Geometry: final body of the model. Coordinates: model frame, mm. A direction names the side the tool comes from. Coordinates: 2 decimals unless noted, no trailing zeros. Order: outer loops, then holes, each group sorted by start corner. A loop starts at its lowest first (then second) coordinate and runs counter-clockwise, first axis right, second up. Notation, with made-up numbers: (-36.5, 45) -> (-16.5, 45) arc R12 cw to (-16.5, 51) -> close; hole circle Ø9 at (63.5, 67.5). An arc over 180 degrees is marked (long way). Use CSV: the item, a comma, the result in double quotes. Start each with the question number.
from build123d import *

# Parameters (mm, degrees)
BOSS_EXTRUDE1_DEPTH = 1.3
BOSS_EXTRUDE3_DEPTH = 3
CUT_EXTRUDE1_DEPTH  = 3
SKETCH11_W          = 6.5
SKETCH11_H          = 9
CUT_EXTRUDE2_DEPTH  = 4.3
SKETCH12_W          = 12.1
SKETCH12_H          = 12.1
CUT_EXTRUDE4_DEPTH  = 1.3
SKETCH17_W          = 14.5
SKETCH17_H          = 14.3
SKETCH17_W_2        = 12.1
SKETCH17_H_2        = 12.1
BOSS_EXTRUDE4_DEPTH = 6.25
CUT_EXTRUDE5_DEPTH  = 4.3
BOSS_EXTRUDE5_DEPTH = 6.25
CUT_EXTRUDE6_START  = -3
CUT_EXTRUDE6_DEPTH  = 23
SKETCH21_W          = 2.5
SKETCH21_H          = 2.5
CUT_EXTRUDE7_DEPTH  = 10
BOSS_EXTRUDE7_DEPTH = 7.6
SKETCH25_W          = 2
SKETCH25_H          = 2
BOSS_EXTRUDE8_DEPTH = 7.6
SKETCH27_W          = 1
SKETCH27_H          = 18.4
CUT_EXTRUDE8_DEPTH  = 7.5
FILLET1_R           = 0.4


with BuildPart() as part:
    # Sketch1 → Boss-Extrude1 (new body)
    with BuildSketch(Plane.XY):
        with BuildLine():
            Line((2.7, 0), (52.9, 0))
            ThreePointArc((52.9, 0), (54.809188309, 0.790811691), (55.6, 2.7))
            Line((55.6, 2.7), (55.6, 19.4))
            ThreePointArc((55.6, 19.4), (54.809188309, 21.309188309), (52.9, 22.1))
            Line((52.9, 22.1), (2.7, 22.1))
            ThreePointArc((2.7, 22.1), (0.790811691, 21.309188309), (0, 19.4))
            Line((0, 19.4), (0, 2.7))
            ThreePointArc((0, 2.7), (0.790811691, 0.790811691), (2.7, 0))
        make_face()
    extrude(amount=BOSS_EXTRUDE1_DEPTH)

    # Sketch4 → Boss-Extrude3 (add)
    with BuildSketch(Plane.XY.offset(1.3)):
        with BuildLine():
            Line((54.25, 2.85), (54.25, 19.25))
            ThreePointArc((54.25, 19.25), (53.810660172, 20.310660172), (52.75, 20.75))
            Line((52.75, 20.75), (2.85, 20.75))
            ThreePointArc((2.85, 20.75), (1.789339828, 20.310660172), (1.35, 19.25))
            Line((1.35, 19.25), (1.35, 2.85))
            ThreePointArc((1.35, 2.85), (1.789339828, 1.789339828), (2.85, 1.35))
            Line((2.85, 1.35), (52.75, 1.35))
            ThreePointArc((52.75, 1.35), (53.810660172, 1.789339828), (54.25, 2.85))
        make_face()
    extrude(amount=BOSS_EXTRUDE3_DEPTH)

    # Sketch5 → Cut-Extrude1 (cut)
    with BuildSketch(Plane.XY.offset(4.3)):
        with BuildLine():
            Line((51.75, 18.75), (3.85, 18.75))
            ThreePointArc((3.85, 18.75), (3.496446609, 18.603553391), (3.35, 18.25))
            Line((3.35, 18.25), (3.35, 3.85))
            ThreePointArc((3.35, 3.85), (3.496446609, 3.496446609), (3.85, 3.35))
            Line((3.85, 3.35), (51.75, 3.35))
            ThreePointArc((51.75, 3.35), (52.103553391, 3.496446609), (52.25, 3.85))
            Line((52.25, 3.85), (52.25, 18.25))
            ThreePointArc((52.25, 18.25), (52.103553391, 18.603553391), (51.75, 18.75))
        make_face()
    extrude(amount=-CUT_EXTRUDE1_DEPTH, mode=Mode.SUBTRACT)

    # Sketch10 → Cut-Revolve1 (revolve, cut)
    with BuildSketch(Plane(origin=(0, 20.75, 0), x_dir=(1, 0, 0), z_dir=(0, 1, 0))):
        with BuildLine():
            Line((40.35, -2), (40.35, -3.6))
            ThreePointArc((40.35, -3.6), (39.55, -2.8), (40.35, -2))
        make_face()
    cut_revolve1 = revolve(axis=Axis((40.35, 20.75, 2), (0, 0, 1)), mode=Mode.SUBTRACT)

    # Mirror1: Cut-Revolve1 across plane
    add(cut_revolve1.mirror(Plane(origin=(0, 11.05, 0), x_dir=(0, 0, 1), z_dir=(0, -1, 0))), mode=Mode.SUBTRACT)

    # Sketch11 → Cut-Extrude2 (cut)
    with BuildSketch(Plane(origin=(0, 0, 0), x_dir=(-1, 0, 0), z_dir=(0, 0, -1))):
        with Locations((-5.8, 7.55)):
            Rectangle(SKETCH11_W, SKETCH11_H)
    extrude(amount=-CUT_EXTRUDE2_DEPTH, mode=Mode.SUBTRACT)

    # Sketch12 → Cut-Extrude4 (cut)
    with BuildSketch(Plane(origin=(0, 0, 0), x_dir=(-1, 0, 0), z_dir=(0, 0, -1))):
        with Locations((-19.75, 10.6)):
            Rectangle(SKETCH12_W, SKETCH12_H)
    extrude(amount=-CUT_EXTRUDE4_DEPTH, mode=Mode.SUBTRACT)

    # Sketch17 → Boss-Extrude4 (add)
    with BuildSketch(Plane(origin=(0, 0, 0), x_dir=(-1, 0, 0), z_dir=(0, 0, -1))):
        with Locations((-19.75, 10.5)):
            Rectangle(SKETCH17_W, SKETCH17_H)
        with Locations((-19.75, 10.6)):
            Rectangle(SKETCH17_W_2, SKETCH17_H_2, mode=Mode.SUBTRACT)
    extrude(amount=-BOSS_EXTRUDE4_DEPTH)

    # Sketch13 → Cut-Extrude5 (cut)
    with BuildSketch(Plane(origin=(0, 0, 0), x_dir=(-1, 0, 0), z_dir=(0, 0, -1))):
        Polygon((-45.055992052, 11.05), (-36.5, 2.494007948), (-27.944007948, 11.05), (-36.5, 19.605992052), align=None)
    extrude(amount=-CUT_EXTRUDE5_DEPTH, mode=Mode.SUBTRACT)

    # Sketch18 → Boss-Extrude5 (add)
    with BuildSketch(Plane(origin=(0, 0, 0), x_dir=(-1, 0, 0), z_dir=(0, 0, -1))):
        Polygon((-46.753048327, 11.05), (-36.5, 0.796951673), (-26.246951673, 11.05), (-36.5, 21.303048327), align=None)
        Polygon((-36.5, 19.605992052), (-45.055992052, 11.05), (-36.5, 2.494007948), (-27.944007948, 11.05), align=None, mode=Mode.SUBTRACT)
    extrude(amount=-BOSS_EXTRUDE5_DEPTH)

    # Sketch20 → Cut-Extrude6 (cut)
    with BuildSketch(Plane.XY.offset(4.3).offset(CUT_EXTRUDE6_START)):
        Polygon((35.946951673, 20.75), (37.053048327, 20.75), (36.5, 21.303048327), align=None)
    cut_extrude6 = extrude(amount=CUT_EXTRUDE6_DEPTH, mode=Mode.SUBTRACT)

    # Mirror2: Cut-Extrude6 across plane
    add(cut_extrude6.mirror(Plane(origin=(0, 11.05, 0), x_dir=(0, 0, 1), z_dir=(0, -1, 0))), mode=Mode.SUBTRACT)

    # Sketch21 → Cut-Extrude7 (cut)
    with BuildSketch(Plane(origin=(0, 0, 0), x_dir=(-1, 0, 0), z_dir=(0, 0, -1))):
        with Locations((-29, 17.1)):
            Rectangle(SKETCH21_W, SKETCH21_H)
    extrude(amount=-CUT_EXTRUDE7_DEPTH, mode=Mode.SUBTRACT)

    # Mirror3: Cut-Revolve1 across plane
    add(cut_revolve1.mirror(Plane.ZY.offset(-27.8)), mode=Mode.SUBTRACT)

    # Mirror3 copy 1 sketch → Mirror3 copy 1 (revolve, cut)
    with BuildSketch(Plane(origin=(55.6, 1.35, 0), x_dir=(-1, 0, 0), z_dir=(0, -1, 0))):
        with BuildLine():
            Line((40.35, -2), (40.35, -3.6))
            ThreePointArc((40.35, -3.6), (39.55, -2.8), (40.35, -2))
        make_face()
    revolve(axis=Axis((15.25, 1.35, 2), (0, 0, 1)), mode=Mode.SUBTRACT)

    # Sketch24 → Boss-Extrude7 (add)
    with BuildSketch(Plane.XY.offset(1.3)):
        Polygon((33.946951673, 3.35), (27, 3.35), (27, 5.85), (31.446951673, 5.85), align=None)
    extrude(amount=BOSS_EXTRUDE7_DEPTH)

    # Sketch25 → Boss-Extrude8 (add)
    with BuildSketch(Plane.XY.offset(1.3)):
        with Locations((43.3, 4.35)):
            Rectangle(SKETCH25_W, SKETCH25_H)
    boss_extrude8 = extrude(amount=BOSS_EXTRUDE8_DEPTH)

    # Mirror4: Boss-Extrude8 across plane
    add(boss_extrude8.mirror(Plane(origin=(0, 11.05, 0), x_dir=(0, 0, 1), z_dir=(0, -1, 0))))

    # Sketch27 → Cut-Extrude8 (cut)
    with BuildSketch(Plane(origin=(54.25, 0, 0), x_dir=(0, 0, -1), z_dir=(1, 0, 0))):
        with Locations((-3.8, 11.05)):
            Rectangle(SKETCH27_W, SKETCH27_H)
    extrude(amount=-CUT_EXTRUDE8_DEPTH, mode=Mode.SUBTRACT)

    # Fillet1
    fillet1_edges = [part.edges().sort_by_distance(p)[0] for p in [
        (36.5, 19.605992052, 3.125),
        (36.5, 2.494007948, 3.125),
    ]]
    fillet(fillet1_edges, radius=FILLET1_R)


solid = part.part
(1) Section A-A (z = 8.25). Return loops of the section in (x, y).
(2) Mould query, pull axis Y, two halves, no side actions, for faces 6 (the face through (28, 22.1, 1)), 7 (the face through (46.75, 20, 4)), 8 (the face through (43, 4, 8.9)). Classes: pulls with the +Y half, pulls with the -Y half, needs draft (parallel to the pull), parting line crosses it, or undercut.
(3) First-contact query: pin 1 (1.3 mm diameter, centred on y = 8.5, z = 4.5, fed in from +X); pin 2 (1 mm diameter, centred on y = 9.5, z = 2.5, fed in from -X); pin 3 (5 mm diameter, centred on x = 10.5, z = 5.5, fed in from -Y). Flat tips, straight axial feed; report the tip coordinate or a pass-through.
(4) Section C-C (x = 50). Return loops of the section in (y, z), then the cut area to 3 significant figures.
(5) Section D-D (y = 15). Return loops of the section in (x, z), then the cut area to 3 significant figures.
(6) Line query: line 1 (Y direction, x = 24.5, z = 3); line 2 (X direction, y = 3.25, z = 2.75); line 3 (X direction, y = 7, z = 2). Output: solid intervals per line, ascending. Write a range as from..to.
(7) Access query for faces 1 (the face through (52.25, 11, 2)), 2 (the face through (53.82, 20.3, 2.45)), 3 (the face through (50, 1.85, 4)), 4 (the face through (27, 5, 8)), 5 (the face through (32.023, 15.129, 3.081)). Directions: +Z, -Z, +X, -X, +Y, -Y. A direction counts if a zero-diameter tool reaches every point of the face in a straight line with its end or side. Return the directions, or none.
(8) Section B-B (x = 18.5). Return loops of the section in (y, z).
Check sheet entries:
1,outline,"(27, 3.35) -> (33.95, 3.35) -> (31.45, 5.85) -> (27, 5.85) -> close; (42.3, 3.35) -> (44.3, 3.35) -> (44.3, 5.35) -> (42.3, 5.35) -> close; (42.3, 16.75) -> (44.3, 16.75) -> (44.3, 18.75) -> (42.3, 18.75) -> close"
2,face 6,"pulls with the +Y half"
2,face 7,"undercut"
2,face 8,"needs draft"
3,pin 1,"stops at x = 44.85"
3,pin 2,"stops at x = 1.35"
3,pin 3,"stops at y = 1.35"
4,outline,"(0, 0) -> (22.1, 0) -> (22.1, 1.3) -> (20.75, 1.3) -> (20.75, 4.3) -> (20.25, 4.3) -> (20.25, 3.3) -> (18.75, 3.3) -> (18.75, 1.3) -> (3.35, 1.3) -> (3.35, 3.3) -> (1.85, 3.3) -> (1.85, 4.3) -> (1.35, 4.3) -> (1.35, 1.3) -> (0, 1.3) -> close"
4,area,"37.7 mm^2"
5,outline,"(0, 0) -> (13.7, 0) -> (13.7, 6.25) -> (12.5, 6.25) -> (12.5, 1.3) -> (3.35, 1.3) -> (3.35, 4.3) -> (1.35, 4.3) -> (1.35, 1.3) -> (0, 1.3) -> close; (25.8, 0) -> (31.89, 0) -> (31.89, 6.25) -> (30.2, 6.25) -> (30.2, 1.3) -> (27, 1.3) -> (27, 6.25) -> (25.8, 6.25) -> close; (41.11, 0) -> (55.6, 0) -> (55.6, 1.3) -> (54.25, 1.3) -> (54.25, 3.3) -> (52.25, 3.3) -> (52.25, 1.3) -> (42.8, 1.3) -> (42.8, 6.25) -> (41.11, 6.25) -> close"
5,area,"83.3 mm^2"
6,line 1,"y = 1.35..4.55, 16.65..17.65, 18.75..20.75"
6,line 2,"x = 1.35..2.55, 9.05..35.74, 37.26..54.25"
6,line 3,"x = 1.35..2.55, 12.5..13.7, 25.8..27, 30.3..31.99, 41.01..42.7, 52.25..54.25"
7,face 1,"+Z"
7,face 2,"+Z, +X, +Y"
7,face 3,"+Z, +X"
7,face 4,"+Z, -X, +Y, -Y"
7,face 5,"+Z, -Z"
8,outline,"(0, 0) -> (4.55, 0) -> (4.55, 6.25) -> (3.35, 6.25) -> (3.35, 4.3) -> (1.35, 4.3) -> (1.35, 1.3) -> (0, 1.3) -> close; (16.65, 0) -> (22.1, 0) -> (22.1, 1.3) -> (20.75, 1.3) -> (20.75, 4.3) -> (18.75, 4.3) -> (18.75, 1.3) -> (17.65, 1.3) -> (17.65, 6.25) -> (16.65, 6.25) -> close"
